Design review of the part built by this model. Coordinates are the model's own, in mm. Face numbers are marked on the shaded views. A direction names the side the tool comes from. Round coordinates to 2 decimals unless told otherwise and drop trailing zeros. Loops run counter-clockwise (first coordinate to the right, second up) from the corner with the lowest first, then second, coordinate; pieces in that order, holes last. Notation, with made-up numbers: M 42,38.25 L 63,38.25 A12 ccw 63,58.25 Z; hole C -32.75,86 d7. An arc over 180 degrees is marked long. One line per item, written item: value. Start each with the question number.
Item 1: We need section C-C (y = 3). Write out the cut boundary in (x, z), then the cut area to 3 significant figures.
Item 2: Clearance check with flat-ended pins moving along their axes: pin 1 (1 mm diameter, centred on y = -1.5, z = -0.5, fed in from -X); pin 2 (9.5 mm diameter, centred on x = -48.5, y = -10, fed in from -Z); pin 3 (8.5 mm diameter, centred on x = 46, y = -5.5, fed in from +Z). State where each tip first meets the part, or that it passes through.
Item 3: Mouldability with a two-part tool opening along X and no side actions: class the marked faces 5, 6, 7 and 8 as released by +X, released by -X, zero draft, split by the parting line, or undercut.
Item 4: For line 1 along X through (y, z) = (-8.75, 6); line 2 along Z through (x, y) = (50.5, -14.75), list the stretches that pass through material, from the lowest coordinate up.
Item 5: We need section A-A (y = -12). Write out the cut boundary in (x, z), then the cut area to 3 significant figures.
Item 6: We need section B-B (x = -48). Write out the cut boundary in (y, z), then the cut area to 3 significant figures.
Item 7: We need section D-D (z = 9.5). Write out the cut boundary in (x, y).
Item 8: For the marked faces 1, 2, 3 and 4, list the 3-axis set-ups (+Z, -Z, +X, -X, +Y, -Y) from which the entire face can be reached by the end or side of a thin tool; tool diameter is ignored.
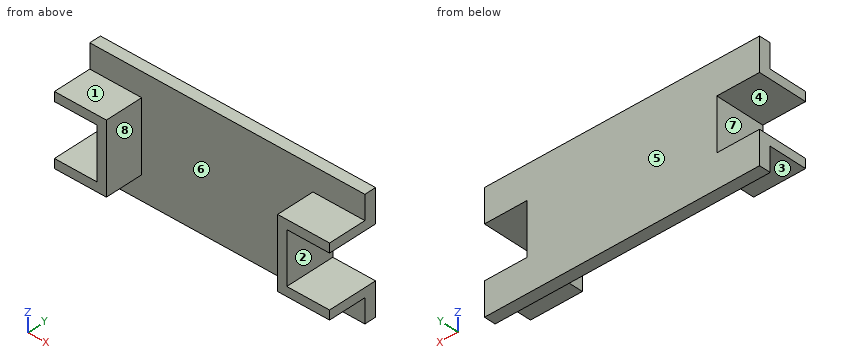
from build123d import *

# Parameters (mm, degrees)
BOSS_EXTRUDE1_DEPTH = 5
BOSS_EXTRUDE2_DEPTH = 16.532


with BuildPart() as part:
    # Sketch1 → Boss-Extrude1 (new body)
    with BuildSketch(Plane(origin=(0, 0, 0), x_dir=(1, 0, 0), z_dir=(0, 1, 0))):
        Polygon((-60, 25.6535), (-60, 11.24975), (-41.343, 11.24975), (-41.343, -11.24975), (-60, -11.24975), (-60, -25.6535), (60, -25.6535), (60, -11.2535), (41.343, -11.2535), (41.343, 11.2535), (60, 11.2535), (60, 25.6535), align=None)
    extrude(amount=BOSS_EXTRUDE1_DEPTH)

    # Sketch2 → Boss-Extrude2 (add)
    with BuildSketch(Plane.XZ):
        Polygon((60, 15.2535), (37.343, 15.2535), (37.343, -15.2535), (60, -15.2535), (60, -11.2535), (41.343, -11.2535), (41.343, 11.2535), (60, 11.2535), align=None)
        Polygon((-60, 11.24975), (-60, 15.24975), (-37.343, 15.24975), (-37.343, -15.2535), (-60, -15.2535), (-60, -11.24975), (-41.343, -11.24975), (-41.343, 11.24975), align=None)
    extrude(amount=BOSS_EXTRUDE2_DEPTH)


solid = part.part
A:
1. outline: M -60,-25.65 L 60,-25.65 L 60,-11.25 L 41.34,-11.25 L 41.34,11.25 L 60,11.25 L 60,25.65 L -60,25.65 L -60,11.25 L -41.34,11.25 L -41.34,-11.25 L -60,-11.25 Z
1. area: 5,320 mm2
2. pin 1: x = -41.34
2. pin 2: z = -15.25
2. pin 3: z = 15.25
3. face 5: zero draft
3. face 6: undercut
3. face 7: released by -X
3. face 8: undercut
4. line 1: -41.34 to -37.34, 37.34 to 41.34
4. line 2: -15.25 to -11.25, 11.25 to 15.25
5. outline: M -60,-15.25 L -37.34,-15.25 L -37.34,15.25 L -60,15.25 L -60,11.25 L -41.34,11.25 L -41.34,-11.25 L -60,-11.25 Z; M 37.34,-15.25 L 60,-15.25 L 60,-11.25 L 41.34,-11.25 L 41.34,11.25 L 60,11.25 L 60,15.25 L 37.34,15.25 Z
5. area: 543 mm2
6. outline: M -16.53,-15.25 L 0,-15.25 L 0,-25.65 L 5,-25.65 L 5,-11.25 L -16.53,-11.25 Z; M -16.53,11.25 L 5,11.25 L 5,25.65 L 0,25.65 L 0,15.25 L -16.53,15.25 Z
6. area: 276 mm2
7. outline: M -41.34,-16.53 L -37.34,-16.53 L -37.34,0 L 37.34,0 L 37.34,-16.53 L 41.34,-16.53 L 41.34,5 L -41.34,5 Z
8. face 1: +Z, +X, -X, -Y
8. face 2: +X, +Y, -Y
8. face 3: -Z, +X, -X, -Y
8. face 4: -X, +Y, -Y
